Here's the drawing with two shaded views (mm, measured from the low corner). I have some questions. A direction names the side the tool comes from. Round coordinates to 2 decimals unless told otherwise and drop trailing zeros. Loops run counter-clockwise (first coordinate to the right, second up) from the corner with the lowest first, then second, coordinate; pieces in that order, holes last. Notation, with made-up numbers: (-8, 25.5) -> (22, 25.5) arc R23 cw to (22, 42.5) -> close; hole circle Ø9 at (65.25, 24). An arc over 180 degrees is marked (long way). Use a Markdown table: item, result.
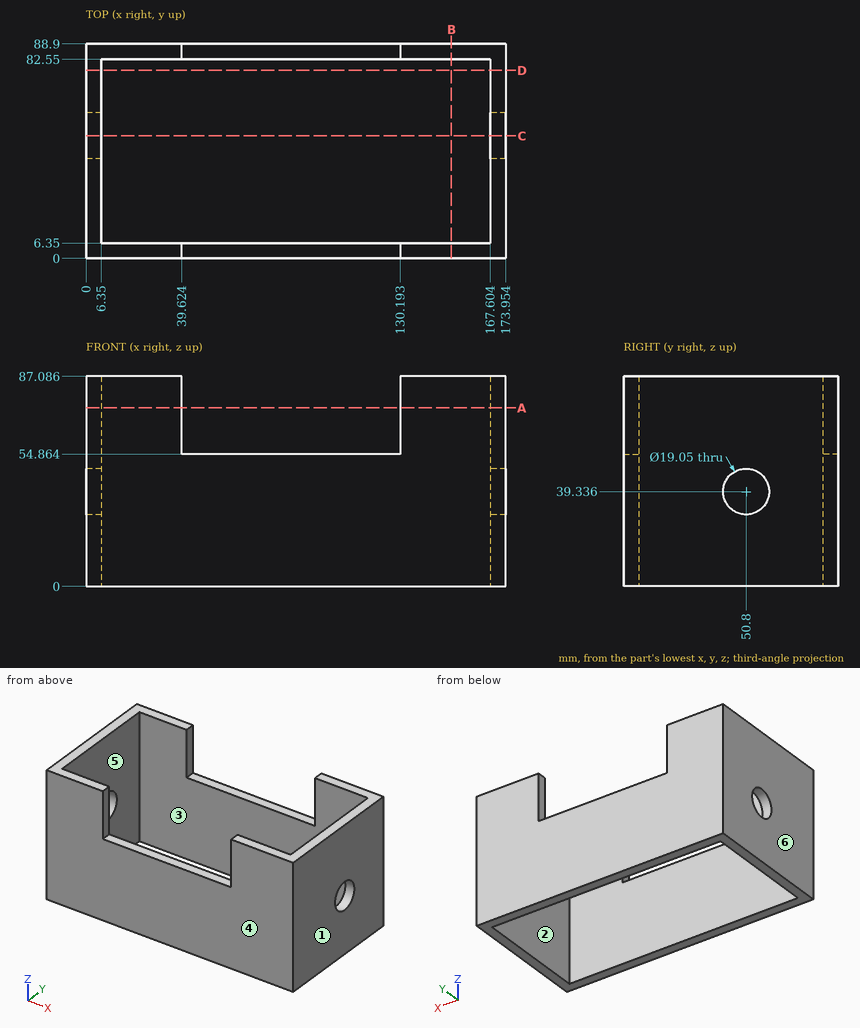
1. I want a section at C-C (y = 50.8). Please give me the cut outline in (x, z).
Answer sheet:
| item | result |
|---|---|
| outline | (0, 0) -> (6.35, 0) -> (6.35, 29.81) -> (0, 29.81) -> close; (0, 48.86) -> (6.35, 48.86) -> (6.35, 87.09) -> (0, 87.09) -> close; (167.6, 0) -> (173.95, 0) -> (173.95, 29.81) -> (167.6, 29.81) -> close; (167.6, 48.86) -> (173.95, 48.86) -> (173.95, 87.09) -> (167.6, 87.09) -> close |
2. I want a section at A-A (z = 74). Please give me the cut outline in (x, y), plus the area to 3 significant figures.
Answer sheet:
| item | result |
|---|---|
| outline | (0, 0) -> (39.62, 0) -> (39.62, 6.35) -> (6.35, 6.35) -> (6.35, 82.55) -> (39.62, 82.55) -> (39.62, 88.9) -> (0, 88.9) -> close; (130.19, 0) -> (173.95, 0) -> (173.95, 88.9) -> (130.19, 88.9) -> (130.19, 82.55) -> (167.6, 82.55) -> (167.6, 6.35) -> (130.19, 6.35) -> close |
| area | 2,030 mm² |
3. Will these pins go through, and if not, where does the flat tip stop? pin 1 Ø3 at (x, y) = (66.5, 84.5) entering from +Z; pin 2 Ø10 at (x, z) = (112, 64) entering from -Y.
Answer sheet:
| item | result |
|---|---|
| pin 1 | stops at z = 54.86 |
| pin 2 | passes through |
4. Which directions (+Z, -Z, +X, -X, +Y, -Y) give clear straight access to the entire face, cutting with the end or side of a thin tool? Please do the marked faces 5 and 6.
Answer sheet:
| item | result |
|---|---|
| face 5 | +Z, -Z |
| face 6 | +Z, -Z, -X, +Y, -Y |
5. I want a section at D-D (y = 78). Please give me the cut outline in (x, z).
Answer sheet:
| item | result |
|---|---|
| outline | (0, 0) -> (6.35, 0) -> (6.35, 87.09) -> (0, 87.09) -> close; (167.6, 0) -> (173.95, 0) -> (173.95, 87.09) -> (167.6, 87.09) -> close |
6. I need wall thicknesses on line 1 (X direction, y = 53.5, z = 28); line 2 (Y direction, x = 93, z = 15); line 3 (Z direction, x = 169.25, y = 50.8). Which ranges of each line are inside material? Lowest first, please.
Answer sheet:
| item | result |
|---|---|
| line 1 | x = 0 to 6.35, 167.6 to 173.95 |
| line 2 | y = 0 to 6.35, 82.55 to 88.9 |
| line 3 | z = 0 to 29.81, 48.86 to 87.09 |
7. If we mould it in two halves opening along X, with no side actions, what happens to the marked faces 1, 2, 3 and 4? For each: +X half, -X half, draft (parallel to the pull), parting line (faces both ways), or undercut.
Answer sheet:
| item | result |
|---|---|
| face 1 | +X half |
| face 2 | undercut |
| face 3 | undercut |
| face 4 | draft |
8. I want a section at B-B (x = 151.5). Please give me the cut outline in (y, z), plus the area to 3 significant figures.
Answer sheet:
| item | result |
|---|---|
| outline | (0, 0) -> (6.35, 0) -> (6.35, 87.09) -> (0, 87.09) -> close; (82.55, 0) -> (88.9, 0) -> (88.9, 87.09) -> (82.55, 87.09) -> close |
| area | 1,110 mm² |
